from build123d import *

# Parameters (mm, degrees)
BASE_FLANGE1_DEPTH      = 15
CUT_EXTRUDE1_DEPTH      = 14
CUT_EXTRUDE1_DEPTH_BACK = 10
SKETCH6_W               = 22.14
SKETCH6_H               = 5
FILLET1_R               = 1
SKETCH7_R               = 2.1
CUT_EXTRUDE2_DEPTH      = 10


# Sheet-metal steps are written as plain solids
with BuildPart() as part:
    # Sketch1 → Base-Flange1 (new body)
    with BuildSketch(Plane(origin=(0, 0, 0), x_dir=(1, 0, 0), z_dir=(0, 1, 0))):
        with BuildLine():
            Line((0, 0), (50, 0))
            ThreePointArc((50, 0), (52.294305745, 7.276608177), (46.241229517, 2.631919427))
            Line((46.241229517, 2.631919427), (41.94683424, 1.068887372))
            ThreePointArc((41.94683424, 1.068887372), (54.91555006, 11.02013302), (50, -4.57))
            Line((50, -4.57), (0, -4.57))
            Line((0, -4.57), (0, 0))
        make_face()
    extrude(amount=BASE_FLANGE1_DEPTH)

    # Sketch6 → Cut-Extrude1 (cut, two sides: drawn at the far end of the back side and taken through both)
    with BuildSketch(Plane(origin=(0, 0, 0), x_dir=(-1, 0, 0), z_dir=(0, 0, -1)).offset(-CUT_EXTRUDE1_DEPTH_BACK)):
        with Locations((-47.5, 7.5)):
            Rectangle(SKETCH6_W, SKETCH6_H)
    extrude(amount=CUT_EXTRUDE1_DEPTH + CUT_EXTRUDE1_DEPTH_BACK, mode=Mode.SUBTRACT)

    # Fillet1
    fillet1_edges = [part.edges().sort_by_distance(p)[0] for p in [
        (41.94683424, 12.5, -1.068887372),
        (0, 15, 2.285),
        (41.94683424, 2.5, -1.068887372),
        (36.43, 5, 2.285),
        (36.43, 10, 2.285),
        (0, 0, 2.285),
    ]]
    fillet(fillet1_edges, radius=FILLET1_R)

    # Sketch7 → Cut-Extrude2 (cut)
    with BuildSketch(Plane(origin=(0, 0, 0), x_dir=(-1, 0, 0), z_dir=(0, 0, -1))):
        with Locations((-21.23, 7.5)):
            Circle(SKETCH7_R)
        with Locations((-33.93, 7.5)):
            Circle(SKETCH7_R)
        with Locations((-8.53, 7.5)):
            Circle(SKETCH7_R)
    extrude(amount=-CUT_EXTRUDE2_DEPTH, mode=Mode.SUBTRACT)


solid = part.part
Geometry: final body of the model. Coordinates: model frame, mm. A direction names the side the tool comes from. Give positions to 0.01 mm unless a question says otherwise; leave off trailing zeros. Loops run counter-clockwise (first coordinate to the right, second up) from the corner with the lowest first, then second, coordinate; pieces in that order, holes last. Notation, with made-up numbers: (24, -22) - (72, -22) arc R18 cw to (72, -6) - close; hole circle Ø8 at (58.25, 38.25). An arc over 180 degrees is marked (long way). One line per question, with ' | ' between items. Start each with the question number.
(1) Contact query for flat-ended pins moving along their axis: pin 1 (1.5 mm diameter, centred on y = 9, z = -0.5, fed in from -X); pin 2 (2.5 mm diameter, centred on x = 33.93, y = 7.5, fed in from +Z); pin 3 (0.9 mm diameter, centred on y = 7, z = 3, fed in from +X); pin 4 (6 mm diameter, centred on y = 7, z = -1, fed in from +X). Output: stop coordinate, or through.
(2) Reachability of faces 1 (the cylindrical face through (36.715, 5.301, 2.253)), 2 (the cylindrical face through (0.285, 0.301, 2.253)), 3 (the cylindrical face through (42.115, 2.535, -1.503)) from +Z, -Z, +X, -X, +Y, -Y: full face, straight path, thin tool, end or side. Return the list, or none.
(3) Ray query, line 1 (Y direction, x = 45, z = 2.5); line 2 (X direction, y = 12.4, z = -4); line 3 (Z direction, x = 50, y = 3.65). Return the intervals inside material, ascending. Write a range as from..to.
(4) Section query C-C on y = 7.5. Return loops of the section in (x, z), then the cut area to 3 significant figures.
(5) Section query B-B on x = 33.93. Return loops of the section in (y, z).
(6) Pull-direction query (X, two-part tool) for faces 4 (the cylindrical face through (34.203, 9.582, 2.253)), 5 (the cylindrical face through (55.136, 12.465, -10.861)), 6 (the flat face through (36.3, 0, 0.4)); classes: released by +X, released by -X, zero draft, split by the parting line, or undercut.
(7) Section query A-A on z = -4. Return loops of the section in (x, y), then the cut area to 3 significant figures.
(8) Section query D-D on z = -9.5. Return loops of the section in (x, y).
The answers:
1) pin 1: x = 0 | pin 2: through | pin 3: x = 36.43 | pin 4: x = 58.54
2) face 1: +Z, -Z, +X | face 2: +Z, -Z, -X, -Y | face 3: +Y, -Y
3) line 1: 0..5, 10..15 | line 2: 41.43..46, 54..58.57 | line 3: -12.57..-8, 0..4.57
4) outline: (0, 0) - (6.43, 0) - (6.43, 4.57) - (0, 4.57) - close; (10.63, 0) - (19.13, 0) - (19.13, 4.57) - (10.63, 4.57) - close; (23.33, 0) - (31.83, 0) - (31.83, 4.57) - (23.33, 4.57) - close; (36.03, 0) - (36.43, 0) - (36.43, 4.57) - (36.03, 4.57) - close | area: 109 mm2
5) outline: (0, 0) - (5.4, 0) - (5.4, 4.57) - (0, 4.57) - close; (9.6, 0) - (15, 0) - (15, 4.57) - (9.6, 4.57) - close
6) face 4: undercut | face 5: split by the parting line | face 6: zero draft
7) outline: (41.43, 0) - (46, 0) - (46, 5) - (41.43, 5) - close; (41.43, 10) - (46, 10) - (46, 15) - (41.43, 15) - close; (54, 0) - (58.57, 0) - (58.57, 5) - (54, 5) - close; (54, 10) - (58.57, 10) - (58.57, 15) - (54, 15) - close | area: 91.4 mm2
8) outline: (43.43, 0) - (56.57, 0) - (56.57, 5) - (43.43, 5) - close; (43.43, 10) - (56.57, 10) - (56.57, 15) - (43.43, 15) - close
